from build123d import *

# Parameters (mm, degrees)
F0_R     = 11.2
F1_DEPTH = 25


with BuildPart() as f1:
    # F0 (on Top) → F1 (new body)
    with BuildSketch(Plane.XY):
        with BuildLine():
            ThreePointArc((0.9477981241, -13.1659287069), (9.6630982412, -8.9924708718), (13.2, 0))
            ThreePointArc((13.2, 0), (9.438299675, 9.2281362823), (0.2971970842, 13.19665389))
            Line((0.2971970842, 13.19665389), (-0.3000556461, 13.1965892036))
            ThreePointArc((-0.3000556461, 13.1965892036), (-13.1956435727, 0.3391027885), (-0.9774661602, -13.1637593379))
            Line((-0.9774661602, -13.1637593379), (0.9477981241, -13.1659287069))
        make_face()
        Circle(F0_R, mode=Mode.SUBTRACT)
        with BuildLine():
            ThreePointArc((0.2971970842, 13.19665389), (9.438299675, 9.2281362823), (13.2, 0))
            ThreePointArc((13.2, 0), (9.6630982412, -8.9924708718), (0.9477981241, -13.1659287069))
            Line((0.9477981241, -13.1659287069), (31.1778370012, -13.1999916203))
            ThreePointArc((31.1778370012, -13.1999916203), (38.5529222641, -10.9575218275), (43.4179762546, -4.9782406771))
            ThreePointArc((43.4179762546, -4.9782406771), (44.3640726701, 0.8690349983), (42.6579258061, 6.5413179718))
            ThreePointArc((42.6579258061, 6.5413179718), (37.8213685594, 11.4149416978), (31.1912809763, 13.1999999226))
            Line((31.1912809763, 13.1999999226), (0.2971970842, 13.19665389))
        make_face()
        with Locations((31.1927106231, 0)):
            Circle(F0_R, mode=Mode.SUBTRACT)
        with BuildLine():
            Line((-0.3000556461, 13.1965892036), (0.2971970842, 13.19665389))
            ThreePointArc((0.2971970842, 13.19665389), (-0.0014296468, 13.1999999226), (-0.3000556461, 13.1965892036))
        make_face()
        with BuildLine():
            ThreePointArc((-0.9774661602, -13.1637593379), (-0.014873622, -13.1999916203), (0.9477981241, -13.1659287069))
            Line((0.9477981241, -13.1659287069), (-0.9774661602, -13.1637593379))
        make_face()
        with BuildLine():
            ThreePointArc((-0.9774661602, -13.1637593379), (-13.1956435727, 0.3391027885), (-0.3000556461, 13.1965892036))
            Line((-0.3000556461, 13.1965892036), (-36.0695777831, 13.192715129))
            Line((-36.0695777831, 13.192715129), (-36.9494019058, 13.1926198383))
            ThreePointArc((-36.9494019058, 13.1926198383), (-42.7568480948, 11.627237838), (-47.2668801052, 7.6477324276))
            ThreePointArc((-47.2668801052, 7.6477324276), (-49.5537048838, 2.0127531993), (-49.0715828762, -4.0494342641))
            ThreePointArc((-49.0715828762, -4.0494342641), (-43.7008466332, -11.0681450441), (-35.1057779137, -13.1253038886))
            Line((-35.1057779137, -13.1253038886), (-0.9774661602, -13.1637593379))
        make_face()
        with Locations((-36.5080609918, 0)):
            Circle(F0_R, mode=Mode.SUBTRACT)
        with BuildLine():
            Line((-36.9494019058, 13.1926198383), (-36.0695777831, 13.192715129))
            ThreePointArc((-36.0695777831, 13.192715129), (-36.5094906386, 13.1999999226), (-36.9494019058, 13.1926198383))
        make_face()
        with BuildLine():
            Line((61.9657859206, 0), (42.6579258061, 6.5413179718))
            ThreePointArc((42.6579258061, 6.5413179718), (44.3640726701, 0.8690349983), (43.4179762546, -4.9782406771))
            Line((43.4179762546, -4.9782406771), (61.9657859206, 0))
        make_face()
        with BuildLine():
            Line((-65.6026080251, 0), (-49.0715828762, -4.0494342641))
            ThreePointArc((-49.0715828762, -4.0494342641), (-49.5537048838, 2.0127531993), (-47.2668801052, 7.6477324276))
            Line((-47.2668801052, 7.6477324276), (-65.6026080251, 0))
        make_face()
    extrude(amount=F1_DEPTH)


solid = f1.part
Source: CAD feature listing. Evaluate the final solid. Frame: model axes, mm. Give positions to 0.01 mm unless a question says otherwise; leave off trailing zeros. Write each loop counter-clockwise with the first axis right and the second up, starting at its lowest first coordinate (ties: lowest second). Pieces come first, ordered by that corner, then holes. Notation, with made-up numbers: M -36,-3.5 L 2,-3.5 A33 ccw 2,35.5 Z; hole C 68.5,88.25 d3. An arc over 180 degrees is marked long. Return JSON: item names as keys, results as strings. Group by question number.
1) Cut plane C-C, the plane x = 5.5. Output: boundary loops of the cut face in (y, z), plus the area to 3 significant figures.
2) Material intervals for line 1 along X through (y, z) = (-10.25, 5.5); line 2 along X through (y, z) = (-5, 3); line 3 along Y through (x, z) = (-11.5, 13), sorted ascending. Write a range as [from, to].
3) Cut plane B-B, the plane y = 2.5. Output: boundary loops of the cut face in (x, z).
4) Cut plane A-A, the plane z = 11.5. Output: boundary loops of the cut face in (x, y).
5) Cut plane D-D, the plane x = -31. Output: boundary loops of the cut face in (y, z), plus the area to 3 significant figures.
6) Pin query (flat end, axial travel): P1, Ø1.5, axis at y = 10.5, z = 13, coming from the -X side; P2, Ø1.5, axis at x = 28, y = -9, coming from the +Z side; P3, Ø8, axis at x = 11, y = 0, coming from the +Z side; P4, Ø1, axis at x = -32, z = 4.5, coming from the +Y side. Return the tip coordinate at first contact, or that it passes through.
7) Pull-direction query (X, two-part tool) for faces 1 (the face through (-11.19, 0.49, 12.32)), 2 (the face through (-3, -12, 25)), 3 (the face through (52.562, -2.524, 12.325)); classes: pulls with the +X half, pulls with the -X half, needs draft (parallel to the pull), parting line crosses it, or undercut.
Recorded:
{
 "1": {"outline": "M -13.17,0 L -9.76,0 L -9.76,25 L -13.17,25 Z; M 9.76,0 L 13.2,0 L 13.2,25 L 9.76,25 Z", "area": "171 mm²"},
 "2": {"line 1": "x = [-44.83, -41.02], [-31.99, -4.51], [4.51, 26.68], [35.71, 39.51]", "line 2": "x = [-48.72, -46.53], [-26.49, -10.02], [10.02, 21.17], [41.21, 43.41]", "line 3": "y = [-13.15, 13.2]"},
 "3": {"outline": "M -59.61,0 L -47.43,0 L -47.43,25 L -59.61,25 Z; M -25.59,0 L -10.92,0 L -10.92,25 L -25.59,25 Z; M 10.92,0 L 20.28,0 L 20.28,25 L 10.92,25 Z; M 42.11,0 L 54.59,0 L 54.59,25 L 42.11,25 Z"},
 "4": {"outline": "M -65.6,0 L -49.07,-4.05 A13.2 ccw -35.11,-13.13 L -0.98,-13.16 A13.2 ccw 0.95,-13.17 L 31.18,-13.2 A13.2 ccw 43.42,-4.98 L 61.97,0 L 42.66,6.54 A13.2 ccw 31.19,13.2 L 0.3,13.2 A13.2 ccw -0.3,13.2 L -36.07,13.19 A13.2 ccw -47.27,7.65 Z; hole C -36.51,0 d22.4; hole C 0,0 d22.4; hole C 31.19,0 d22.4"},
 "5": {"outline": "M -13.13,0 L -9.75,0 L -9.75,25 L -13.13,25 Z; M 9.75,0 L 13.19,0 L 13.19,25 L 9.75,25 Z", "area": "170 mm²"},
 "6": {"P1": "stops at x = -45.41", "P2": "passes through", "P3": "stops at z = 25", "P4": "stops at y = 13.19"},
 "7": {"face 1": "undercut", "face 2": "needs draft", "face 3": "pulls with the +X half"}
}
